```python
from build123d import *

# Parameters (mm, degrees)
F0_W      = 31.19
F0_H      = 12.93
F1_DEPTH  = 1.4
F2_R      = 1.6
F3_DEPTH  = 1.401
F4_R      = 1.5
F5_W      = 8.7
F5_H      = 3.4
F6_DEPTH  = 1.401
F7_W      = 14.75
F7_H      = 8.5
F8_DEPTH  = 21
F9_W      = 10.75
F9_H      = 4.5
F10_DEPTH = 21
F11_R     = 0.9
F12_DEPTH = 10.716


with BuildPart() as f1:
    # F0 (on Top) → F1 (new body)
    with BuildSketch(Plane.XY):
        Rectangle(F0_W, F0_H)
    extrude(amount=F1_DEPTH)

    # F2 (on face) → F3 (cut, through all)
    with BuildSketch(Plane.XY.offset(1.4)):
        with Locations((-12.56, 0)):
            Circle(F2_R)
        with Locations((12.56, 0)):
            Circle(F2_R)
    extrude(amount=-F3_DEPTH, mode=Mode.SUBTRACT)

    # F4
    f4_edges = [f1.edges().sort_by_distance(p)[0] for p in [
        (15.595, -6.465, 0.7),
        (15.595, 6.465, 0.7),
        (-15.595, -6.465, 0.7),
        (-15.595, 6.465, 0.7),
    ]]
    fillet(f4_edges, radius=F4_R)

    # F5 (on face) → F6 (cut, through all)
    with BuildSketch(Plane.XY.offset(1.4)):
        Rectangle(F5_W, F5_H)
    extrude(amount=-F6_DEPTH, mode=Mode.SUBTRACT)

    # F7 (on face) → F8 (join)
    with BuildSketch(Plane.XY.offset(1.4)):
        Rectangle(F7_W, F7_H)
    extrude(amount=F8_DEPTH)

    # F9 (on face) → F10 (cut, through all)
    with BuildSketch(Plane.XY.offset(22.4)):
        Rectangle(F9_W, F9_H)
    extrude(amount=-F10_DEPTH, mode=Mode.SUBTRACT)

    # F11 (on face) → F12 (cut, through all)
    with BuildSketch(Plane.XZ.offset(4.25)):
        with Locations((-4.8, 20.5)):
            Circle(F11_R)
        with Locations((4.8, 20.5)):
            Circle(F11_R)
    extrude(amount=-F12_DEPTH, mode=Mode.SUBTRACT)


solid = f1.part
```
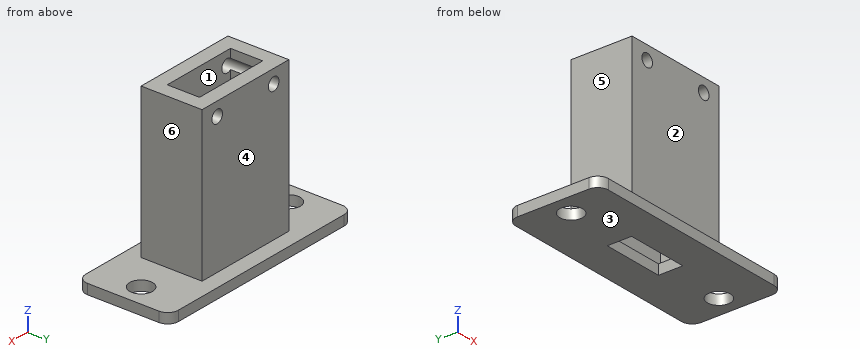
Read the model definition and answer for the solid it produces. Units are mm, in the model's axes. Face numbers are marked on the shaded views. A direction names the side the tool comes from. Coordinates: 2 decimals unless noted, no trailing zeros. Write each loop counter-clockwise with the first axis right and the second up, starting at its lowest first coordinate (ties: lowest second). Pieces come first, ordered by that corner, then holes. Notation, with made-up numbers: (-27.75, -15.75) -> (-9.75, -15.75) arc R19 cw to (-9.75, -7.75) -> close; hole circle Ø4 at (-28.5, 56.25). An arc over 180 degrees is marked (long way). Answer as a JSON object with one key per item and string values.
Q1. The part is cut by section B-B on y = 0. Give the vertices of the cut face in (x, z) (3 decimals).
The answers:
{"outline": "(-15.595, 0) -> (-14.16, 0) -> (-14.16, 1.4) -> (-15.595, 1.4) -> close; (-10.96, 0) -> (-4.35, 0) -> (-4.35, 1.4) -> (-5.375, 1.4) -> (-5.375, 19.808) arc R0.9 cw to (-5.375, 21.192) -> (-5.375, 22.4) -> (-7.375, 22.4) -> (-7.375, 1.4) -> (-10.96, 1.4) -> close; (4.35, 0) -> (10.96, 0) -> (10.96, 1.4) -> (7.375, 1.4) -> (7.375, 22.4) -> (5.375, 22.4) -> (5.375, 21.192) arc R0.9 cw to (5.375, 19.808) -> (5.375, 1.4) -> (4.35, 1.4) -> close; (14.16, 0) -> (15.595, 0) -> (15.595, 1.4) -> (14.16, 1.4) -> close"}
Q2. The part is cut by section D-D on x = -1.5. Give the vertices of the cut face in (y, z) (3 decimals).
The answers:
{"outline": "(-6.465, 0) -> (-1.7, 0) -> (-1.7, 1.4) -> (-2.25, 1.4) -> (-2.25, 22.4) -> (-4.25, 22.4) -> (-4.25, 1.4) -> (-6.465, 1.4) -> close; (1.7, 0) -> (6.465, 0) -> (6.465, 1.4) -> (4.25, 1.4) -> (4.25, 22.4) -> (2.25, 22.4) -> (2.25, 1.4) -> (1.7, 1.4) -> close"}
Q3. Flat-ended cylindrical pins translate along their axes: pin 1 Ø5 at (y, z) = (0.5, 10) entering from +X (3 decimals); pin 2 Ø12 at (x, z) = (-1.5, 15) entering from -Y; pin 3 Ø3 at (x, z) = (-1.5, 12) entering from +Y. Find the tip coordinate at first contact, or state that the pin passes through.
The answers:
{"pin 1": "stops at x = 7.375", "pin 2": "stops at y = -4.25", "pin 3": "stops at y = 4.25"}
Q4. The part is cut by section C-C on z = 20.5. Give the vertices of the cut face in (x, y) (3 decimals), then the cut area to 3 significant figures.
The answers:
{"outline": "(-7.375, -4.25) -> (-5.7, -4.25) -> (-5.7, 4.25) -> (-7.375, 4.25) -> close; (-3.9, -4.25) -> (3.9, -4.25) -> (3.9, -2.25) -> (-3.9, -2.25) -> close; (-3.9, 2.25) -> (3.9, 2.25) -> (3.9, 4.25) -> (-3.9, 4.25) -> close; (5.7, -4.25) -> (7.375, -4.25) -> (7.375, 4.25) -> (5.7, 4.25) -> close", "area": "59.7 mm2"}
Q5. The part is cut by section A-A on x = -4.8. Give the vertices of the cut face in (y, z) (3 decimals).
The answers:
{"outline": "(-6.465, 0) -> (6.465, 0) -> (6.465, 1.4) -> (4.25, 1.4) -> (4.25, 19.6) -> (2.25, 19.6) -> (2.25, 1.4) -> (-2.25, 1.4) -> (-2.25, 19.6) -> (-4.25, 19.6) -> (-4.25, 1.4) -> (-6.465, 1.4) -> close; (-4.25, 21.4) -> (-2.25, 21.4) -> (-2.25, 22.4) -> (-4.25, 22.4) -> close; (2.25, 21.4) -> (4.25, 21.4) -> (4.25, 22.4) -> (2.25, 22.4) -> close"}
Q6. Consider line 1 (Y direction, x = -4, z = 4.5); line 2 (X direction, y = 0.75, z = 12.5) (3 decimals); line 3 (Y direction, x = 12.56, z = 0.5) (3 decimals). Determine where each line is inside the solid, lowest interval first. Write a range as [from, to].
The answers:
{"line 1": "y = [-4.25, -2.25], [2.25, 4.25]", "line 2": "x = [-7.375, -5.375], [5.375, 7.375]", "line 3": "y = [-6.465, -1.6], [1.6, 6.465]"}
Q7. Determine the mould class of the marked faces 1, 2 and 3 for opening direction Y: pulls with the +Y half, pulls with the -Y half, needs draft (parallel to the pull), parting line crosses it, or undercut.
The answers:
{"face 1": "undercut", "face 2": "pulls with the -Y half", "face 3": "needs draft"}
Q8. A tool of negligible diameter and unlimited length cuts with its end or side. For the marked faces 4, 5 and 6, from which of +Z, -Z, +X, -X, +Y, -Y can it reach the whole face along a straight path? Write none if from no direction.
The answers:
{"face 4": "+Z, +X, -X, +Y", "face 5": "+Z, -X, +Y, -Y", "face 6": "+Z, +X, +Y, -Y"}
